Source: CAD feature listing. Evaluate the final solid. Frame: model axes, mm. A direction names the side the tool comes from. Give positions to 0.01 mm unless a question says otherwise; leave off trailing zeros. Order: outer loops, then holes, each group sorted by start corner. A loop starts at its lowest first (then second) coordinate and runs counter-clockwise, first axis right, second up. Notation, with made-up numbers: (73.25, -18.75) - (102.25, -18.75) arc R21 cw to (102.25, 10.25) - close; hole circle Ø7 at (4, -7). An arc over 180 degrees is marked (long way). Use CSV: the item, a comma, the result in double quotes.
```python
from build123d import *

# Parameters (mm, degrees)
SKETCH1_W                       = 400
SKETCH1_H                       = 100
BASE_DEPTH                      = 12
PART_TAPE_MOVER_CUTOUT_DEPTH    = 207.504237245
PRESS_PLATE_CUTOUT_DEPTH        = 207.504237245
ROLLER_CUTOUT_DEPTH             = 207.504237245
SKETCH5_W                       = 315.5
SKETCH5_H                       = 8
PART_TAPE_CUTOUT_DEPTH          = 5.5
SKETCH6_W                       = 315.5
SKETCH6_H                       = 12
PART_TAPE_REST_DEPTH            = 1
CBORE_FOR_M6_SHCS1_AT_2_COUNT   = 2
CBORE_FOR_M6_SHCS1_AT_2_PITCH   = 240
CBORE_FOR_M6_SHCS1_AT_3_COUNT   = 2
CBORE_FOR_M6_SHCS1_AT_3_PITCH   = 252.982212813
LPATTERN2_COUNT                 = 2
LPATTERN2_PITCH                 = 14
LPATTERN2_COUNT_DIR2            = 2
LPATTERN2_PITCH_DIR2            = 50
M5X0_8_TAPPED_HOLE1_D           = 4.2
M5X0_8_TAPPED_HOLE1_DEPTH       = 10
M5X0_8_TAPPED_HOLE1_CSINK_D     = 5.05
M5X0_8_TAPPED_HOLE1_CSINK_ANGLE = 90
M5X0_8_TAPPED_HOLE1_TIP         = 1.2618073
M4X0_7_TAPPED_HOLE1_D           = 3.3
M4X0_7_TAPPED_HOLE1_DEPTH       = 10.1
M4X0_7_TAPPED_HOLE1_CSINK_D     = 4.05
M4X0_7_TAPPED_HOLE1_CSINK_ANGLE = 90
M4X0_7_TAPPED_HOLE1_TIP         = 0.991420021
M3X0_5_TAPPED_HOLE1_D           = 2.5
M3X0_5_TAPPED_HOLE1_CSINK_D     = 3.05
M3X0_5_TAPPED_HOLE1_CSINK_ANGLE = 90
M5X0_8_TAPPED_HOLE2_D           = 4.2
M5X0_8_TAPPED_HOLE2_CSINK_D     = 5.05
M5X0_8_TAPPED_HOLE2_CSINK_ANGLE = 90
M4X0_7_TAPPED_HOLE2_D           = 3.3
M4X0_7_TAPPED_HOLE2_CSINK_D     = 4.05
M4X0_7_TAPPED_HOLE2_CSINK_ANGLE = 90
CBORE_SLOT_FOR_M5_SHCS2_DEPTH   = 12
CBORE_START                     = 7
CBORE_SLOT_FOR_M5_SHCS2_2_DEPTH = 5
LPATTERN3_COUNT                 = 2
LPATTERN3_PITCH                 = 83.75
LPATTERN3_COUNT_DIR2            = 2
LPATTERN3_PITCH_DIR2            = 40


# Read off the part's stored shape, not the designer's step: CBORE SLOT for M5 SHCS2
with BuildPart() as part:
    # Sketch1 → Base (new body)
    with BuildSketch(Plane.XY):
        Rectangle(SKETCH1_W, SKETCH1_H)
    extrude(amount=BASE_DEPTH)

    # Sketch2 → Part Tape Mover Cutout (cut, through all)
    with BuildSketch(Plane.XY.offset(12)):
        with BuildLine():
            Line((200, 0), (149, 0))
            ThreePointArc((149, 0), (146.525126266, 1.025126266), (145.5, 3.5))
            Line((145.5, 3.5), (145.5, 36.5))
            ThreePointArc((145.5, 36.5), (146.525126266, 38.974873734), (149, 40))
            Line((149, 40), (200, 40))
            Line((200, 40), (200, 0))
        make_face()
    extrude(amount=-PART_TAPE_MOVER_CUTOUT_DEPTH, mode=Mode.SUBTRACT)

    # Sketch3 → Press Plate Cutout (cut, through all)
    with BuildSketch(Plane.XY.offset(12)):
        with BuildLine():
            Line((41.5, -10), (103.5, -10))
            ThreePointArc((103.5, -10), (105.974873734, -8.974873734), (107, -6.5))
            Line((107, -6.5), (107, 50))
            Line((107, 50), (38, 50))
            Line((38, 50), (38, -6.5))
            ThreePointArc((38, -6.5), (39.025126266, -8.974873734), (41.5, -10))
        make_face()
    extrude(amount=-PRESS_PLATE_CUTOUT_DEPTH, mode=Mode.SUBTRACT)

    # Sketch4 → Roller Cutout (cut, through all)
    with BuildSketch(Plane.XY.offset(12)):
        with BuildLine():
            Line((-200, 40), (-173.5, 40))
            ThreePointArc((-173.5, 40), (-171.025126266, 38.974873734), (-170, 36.5))
            Line((-170, 36.5), (-170, 3.5))
            ThreePointArc((-170, 3.5), (-171.025126266, 1.025126266), (-173.5, 0))
            Line((-173.5, 0), (-200, 0))
            Line((-200, 0), (-200, 40))
        make_face()
    extrude(amount=-ROLLER_CUTOUT_DEPTH, mode=Mode.SUBTRACT)

    # Sketch5 → Part Tape Cutout (cut)
    with BuildSketch(Plane.XY.offset(12)):
        with Locations((-12.25, 19)):
            Rectangle(SKETCH5_W, SKETCH5_H)
    extrude(amount=-PART_TAPE_CUTOUT_DEPTH, mode=Mode.SUBTRACT)

    # Sketch6 → Part Tape Rest (cut)
    with BuildSketch(Plane.XY.offset(12)):
        with Locations((-12.25, 18)):
            Rectangle(SKETCH6_W, SKETCH6_H)
    extrude(amount=-PART_TAPE_REST_DEPTH, mode=Mode.SUBTRACT)

    # Sketch16 → CBORE for M6 SHCS1 (revolve, cut)
    with BuildSketch(Plane(origin=(190, -40, 12), x_dir=(0, -1, 0), z_dir=(1, 0, 0))):
        Polygon((0, 0), (0, 12), (3.3, 12), (3.3, 6), (5.5, 6), (5.5, 0.025), (5.525, 0), align=None)
    cbore_for_m6_shcs1 = revolve(axis=Axis((190, -40, 18.35), (0, 0, -1)), mode=Mode.SUBTRACT)

    # CBORE for M6 SHCS1 at 2: CBORE for M6 SHCS1 ×2
    with Locations(*[(-i * CBORE_FOR_M6_SHCS1_AT_2_PITCH, 0, 0) for i in range(1, CBORE_FOR_M6_SHCS1_AT_2_COUNT)]):
        add(cbore_for_m6_shcs1, mode=Mode.SUBTRACT)

    # CBORE for M6 SHCS1 at 3: CBORE for M6 SHCS1 ×2
    with Locations(*[Vector(-0.9486832980505139, 0.316227766016838, 0) * (i * CBORE_FOR_M6_SHCS1_AT_3_PITCH) for i in range(1, CBORE_FOR_M6_SHCS1_AT_3_COUNT)]):
        add(cbore_for_m6_shcs1, mode=Mode.SUBTRACT)

    # Sketch18 → CBORE for M3 SHCS2 (revolve, cut)
    with BuildSketch(Plane(origin=(-195, 45, 12), x_dir=(0, -1, 0), z_dir=(1, 0, 0))):
        Polygon((0, 0), (0, 12), (1.7, 12), (1.7, 3), (3.25, 3), (3.25, 0.025), (3.275, 0), align=None)
    cbore_for_m3_shcs2 = revolve(axis=Axis((-195, 45, 18.35), (0, 0, -1)), mode=Mode.SUBTRACT)

    # LPattern2: CBORE for M3 SHCS2 2 × 2
    with Locations(*[(i * LPATTERN2_PITCH, -j * LPATTERN2_PITCH_DIR2, 0) for i in range(LPATTERN2_COUNT) for j in range(LPATTERN2_COUNT_DIR2) if (i, j) != (0, 0)]):
        add(cbore_for_m3_shcs2, mode=Mode.SUBTRACT)

    # M5x0.8 Tapped Hole1
    with Locations(Plane(origin=(0, 50, 0), x_dir=(1, 0, 0), z_dir=(0, 1, 0))):
        with Locations((192, -6), (141, -6), (24, -6), (4, -6)):
            CounterSinkHole(M5X0_8_TAPPED_HOLE1_D / 2, M5X0_8_TAPPED_HOLE1_CSINK_D / 2, depth=M5X0_8_TAPPED_HOLE1_DEPTH, counter_sink_angle=M5X0_8_TAPPED_HOLE1_CSINK_ANGLE)
            with Locations((0, 0, -(M5X0_8_TAPPED_HOLE1_DEPTH + M5X0_8_TAPPED_HOLE1_TIP / 2))):  # 118° drill point
                Cone(0, M5X0_8_TAPPED_HOLE1_D / 2, M5X0_8_TAPPED_HOLE1_TIP, mode=Mode.SUBTRACT)

    # M4x0.7 Tapped Hole1
    with Locations(Plane(origin=(0, 50, 0), x_dir=(1, 0, 0), z_dir=(0, 1, 0))):
        with Locations((-150, -6), (-110, -6)):
            CounterSinkHole(M4X0_7_TAPPED_HOLE1_D / 2, M4X0_7_TAPPED_HOLE1_CSINK_D / 2, depth=M4X0_7_TAPPED_HOLE1_DEPTH, counter_sink_angle=M4X0_7_TAPPED_HOLE1_CSINK_ANGLE)
            with Locations((0, 0, -(M4X0_7_TAPPED_HOLE1_DEPTH + M4X0_7_TAPPED_HOLE1_TIP / 2))):  # 118° drill point
                Cone(0, M4X0_7_TAPPED_HOLE1_D / 2, M4X0_7_TAPPED_HOLE1_TIP, mode=Mode.SUBTRACT)

    # M3x0.5 Tapped Hole1 (through all)
    with Locations(Plane.XY.offset(12)):
        with Locations((-164.15, 40.25), (-117.5, 4.3), (-164.15, 0.25)):
            CounterSinkHole(M3X0_5_TAPPED_HOLE1_D / 2, M3X0_5_TAPPED_HOLE1_CSINK_D / 2, counter_sink_angle=M3X0_5_TAPPED_HOLE1_CSINK_ANGLE)

    # M5x0.8 Tapped Hole2 (through all)
    with Locations(Plane.XY.offset(12)):
        with Locations((-140, 30.25), (-100, 30.25)):
            CounterSinkHole(M5X0_8_TAPPED_HOLE2_D / 2, M5X0_8_TAPPED_HOLE2_CSINK_D / 2, counter_sink_angle=M5X0_8_TAPPED_HOLE2_CSINK_ANGLE)

    # M4x0.7 Tapped Hole2 (through all)
    with Locations(Plane.XY.offset(12)):
        with Locations((8, 32.5), (8, 4)):
            CounterSinkHole(M4X0_7_TAPPED_HOLE2_D / 2, M4X0_7_TAPPED_HOLE2_CSINK_D / 2, counter_sink_angle=M4X0_7_TAPPED_HOLE2_CSINK_ANGLE)

    # CBORE SLOT for M5 SHCS2 outline → CBORE SLOT for M5 SHCS2 (cut)
    with BuildSketch(Plane.XY):
        with BuildLine():
            Line((117.25, 36.25), (117.25, 43.25))
            ThreePointArc((117.25, 43.25), (114.5, 46), (111.75, 43.25))
            Line((111.75, 43.25), (111.75, 36.25))
            ThreePointArc((111.75, 36.25), (114.5, 33.5), (117.25, 36.25))
        make_face()
    cbore_slot_for_m5_shcs2 = extrude(amount=CBORE_SLOT_FOR_M5_SHCS2_DEPTH, mode=Mode.SUBTRACT)

    # CBORE SLOT for M5 SHCS2 2 outline → CBORE SLOT for M5 SHCS2 2 (cut)
    with BuildSketch(Plane.XY.offset(CBORE_START)):
        with BuildLine():
            Line((119.25, 36.25), (119.25, 43.25))
            ThreePointArc((119.25, 43.25), (114.5, 48), (109.75, 43.25))
            Line((109.75, 43.25), (109.75, 36.25))
            ThreePointArc((109.75, 36.25), (114.5, 31.5), (119.25, 36.25))
        make_face()
        with BuildLine():
            ThreePointArc((111.75, 43.25), (114.5, 46), (117.25, 43.25))
            Line((117.25, 43.25), (117.25, 36.25))
            ThreePointArc((117.25, 36.25), (114.5, 33.5), (111.75, 36.25))
            Line((111.75, 36.25), (111.75, 43.25))
        make_face(mode=Mode.SUBTRACT)
    cbore_slot_for_m5_shcs2_2 = extrude(amount=CBORE_SLOT_FOR_M5_SHCS2_2_DEPTH, mode=Mode.SUBTRACT)

    # LPattern3: CBORE SLOT for M5 SHCS2, CBORE SLOT for M5 SHCS2 2 2 × 2
    with Locations(*[(-i * LPATTERN3_PITCH, -j * LPATTERN3_PITCH_DIR2, 0) for i in range(LPATTERN3_COUNT) for j in range(LPATTERN3_COUNT_DIR2) if (i, j) != (0, 0)]):
        add(cbore_slot_for_m5_shcs2, mode=Mode.SUBTRACT)
        add(cbore_slot_for_m5_shcs2_2, mode=Mode.SUBTRACT)


solid = part.part
```
Item 1: First-contact query: pin 1 (5 mm diameter, centred on x = -181, y = 45, fed in from +Z); pin 2 (7.5 mm diameter, centred on x = 31.5, y = 42, fed in from +Z); pin 3 (1.5 mm diameter, centred on y = 1.5, z = 10, fed in from -X). Flat tips, straight axial feed; report the tip coordinate or a pass-through.
Filled in:
pin 1,"stops at z = 9"
pin 2,"stops at z = 7"
pin 3,"stops at x = -171.33"
Item 2: Section A-A on x = -16.5. Return the cut outline in (y, z), then the cut area to 3 significant figures.
Filled in:
outline,"(-50, 0) - (50, 0) - (50, 12) - (24, 12) - (24, 11) - (23, 11) - (23, 6.5) - (15, 6.5) - (15, 11) - (12, 11) - (12, 12) - (-50, 12) - close"
area,"1,150 mm2"
Item 3: Material intervals for line 1 (Y direction, x = -195, z = 10.4); line 2 (Y direction, x = 190, z = 10.6); line 3 (Y direction, x = 8, z = 4.25), sorted ascending. Write a range as from..to.
Filled in:
line 1,"y = -50..-8.25, -1.75..0, 40..41.75, 48.25..50"
line 2,"y = -50..-45.5, -34.5..0, 40..50"
line 3,"y = -50..2.35, 5.65..30.85, 34.15..50"
Item 4: Mould query, pull axis Y, two halves, no side actions, for faces 1 (the flat face through (33.5, 40, 3)), 2 (the flat face through (153, 50, 6)), 3 (the flat face through (200, -25, 6)). Classes: released by +Y, released by -Y, zero draft, split by the parting line, or undercut.
Filled in:
face 1,"undercut"
face 2,"released by +Y"
face 3,"zero draft"
Item 5: Set-up query: faces 4 (the flat face through (174, 40, 6)), 5 (the flat face through (-179.6, -3.6, 9)), 6 (the flat face through (107, 21, 6)), 7 (the flat face through (117.25, 0, 3)). Return all of +Z, -Z, +X, -X, +Y, -Y with unobstructed straight access to the full face (end or side cutting, diameter ignored); none if empty.
Filled in:
face 4,"+Z, -Z, +X"
face 5,"+Z"
face 6,"+Z, -Z, +Y"
face 7,"+Z, -Z"
Item 6: Section C-C on x = 51. Return the cut outline in (y, z), then the cut area to 3 significant figures.
Filled in:
outline,"(-50, 0) - (-10, 0) - (-10, 12) - (-50, 12) - close"
area,"480 mm2"
Item 7: Section B-B on y = 18.5. Return the cut outline in (x, z).
Filled in:
outline,"(-170, 0) - (38, 0) - (38, 6.5) - (-170, 6.5) - close; (107, 0) - (145.5, 0) - (145.5, 6.5) - (107, 6.5) - close"
